Autodesk Inventor part; units mm, degrees
ref_plane "YZ Plane" through (0, 0, 0) normal (1, 0, 0) x (0, 1, 0)
ref_plane "XZ Plane" through (0, 0, 0) normal (0, 1, 0) x (-1, 0, 0)
ref_plane "XY Plane" through (0, 0, 0) normal (0, 0, 1) x (1, 0, 0)
sketch "Sketch1" plane through (0, 0, 0) normal (0, 0, 1) x (1, 0, 0)
  line L0 (-12.1708, 16.0073) -> (13.2292, 16.0073)
  line L1 (13.2292, 16.0073) -> (13.2292, -34.7927)
  line L2 (13.2292, -34.7927) -> (-12.1708, -34.7927)
  line L3 (-12.1708, -34.7927) -> (-12.1708, 16.0073)
  line L4 (11.9592, 14.7373) -> (-10.9008, 14.7373)
  line L5 (-10.9008, 14.7373) -> (-10.9008, -33.5227)
  line L6 (-10.9008, -33.5227) -> (11.9592, -33.5227)
  line L7 (11.9592, -33.5227) -> (11.9592, 14.7373)
  point P0 (0, 0)
  dimension "d0" = 25.4
  dimension "d1" = 50.8
  dimension "d2" = 1.27
extrude "Extrusion1" add sketch "Sketch1" along normal blind 762
sketch "Sketch2" plane through (-12.1708, 16.0073, 0) normal (0, 1, 0) x (1, 0, 0)
  circle A0 centre (12.7, -12.7) radius 1.7272
  line L0 (25.4, 0) -> (0, 0)
  line L1 (0, 0) -> (0, -762)
  point P0 (12.1708, 0)
  dimension "d5" = 3.4544
  dimension "d6" = 12.7
  dimension "d7" = 12.7
extrude "Extrusion2" cut sketch "Sketch2" against normal through all
pattern_linear "Rectangular Pattern1" count 30 spacing 25.4 along (0, 0, 1) of "Extrusion2"
equation "\"d3\" = d13"
equation "\"d13\" = 762"
properties part number "VerseFrame 30in"
The model under review builds one solid part; all positions refer to its coordinate system, in mm. A direction names the side the tool comes from. Give positions to 0.01 mm unless a question says otherwise; leave off trailing zeros. Order: outer loops, then holes, each group sorted by start corner. A loop starts at its lowest first (then second) coordinate and runs counter-clockwise, first axis right, second up. Notation, with made-up numbers: M -33.5,-17 L -3.5,-17 A32 cw -3.5,12 Z; hole C -38.5,33 d10. An arc over 180 degrees is marked long. One line per question, with ' | ' between items. Start each with the question number.
1) Mouldability with a two-part tool opening along Y and no side actions: class faces 3 (the face through (0, 16.007, 376)), 4 (the face through (13.229, -9, 376)), 5 (the face through (1, 14.737, 376)) as pulls with the +Y half, pulls with the -Y half, needs draft (parallel to the pull), parting line crosses it, or undercut.
2) Wall thickness on L1, parallel to Y at x = 4.25, z = 120; L2, parallel to X at y = -22, z = 45.5; L3, parallel to X at y = -33.9, z = 292.1: over which ranges is each line inside the solid? List them lowest first. Write a range as from..to.
3) Consider section B-B, the plane x = -6.75. Give the boundary of the cut face in (y, z).
4) Clearance check with a flat-ended pin moving along its axis: P1, Ø2, axis at x = 0.53, z = 292.1, coming from the +Y side. State where the tip first meets the part, or that it passes through.
5) Consider section A-A, the plane y = -7. Give the boundary of the cut face in (x, z).
6) For faces 1 (the face through (-12, -9, 762)), 2 (the face through (0, -33.523, 376)), list the 3-axis set-ups (+Z, -Z, +X, -X, +Y, -Y) from which the entire face can be reached by the end or side of a thin tool; tool diameter is ignored.
Found:
1) face 3: pulls with the +Y half | face 4: needs draft | face 5: undercut
2) L1: y = -34.79..-33.52, 14.74..16.01 | L2: x = -12.17..-10.9, 11.96..13.23 | L3: x = -12.17..-1.2, 2.26..13.23
3) outline: M -34.79,0 L -33.52,0 L -33.52,762 L -34.79,762 Z; M 14.74,0 L 16.01,0 L 16.01,762 L 14.74,762 Z
4) P1: passes through
5) outline: M -12.17,0 L -10.9,0 L -10.9,762 L -12.17,762 Z; M 11.96,0 L 13.23,0 L 13.23,762 L 11.96,762 Z
6) face 1: +Z, +X, -X, +Y, -Y | face 2: +Z, -Z
